Part model, mm, in its own coordinate system. Face numbers are marked on the shaded views. A direction names the side the tool comes from. Coordinates: 2 decimals unless noted, no trailing zeros. Order: outer loops, then holes, each group sorted by start corner. A loop starts at its lowest first (then second) coordinate and runs counter-clockwise, first axis right, second up.
from build123d import *

# Parameters (mm, degrees)
SKETCH1_W                  = 43.18
SKETCH1_H                  = 50.927
BOSS_EXTRUDE1_DEPTH        = 5.08
BOSS_EXTRUDE2_DEPTH        = 2.286
BOSS_EXTRUDE3_DEPTH        = 2.286
SKETCH4_W                  = 43.18
SKETCH4_H                  = 50.927
CUT_EXTRUDE1_DEPTH         = 2.794
BOSS_EXTRUDE4_DEPTH        = 2.54
SKETCH6_W                  = 63.373
SKETCH6_H                  = 2.286
BOSS_EXTRUDE5_DEPTH        = 27.813
SKETCH7_W                  = 25.273
SKETCH7_H                  = 63.373
BOSS_EXTRUDE6_DEPTH        = 12.7
SKETCH8_W                  = 63.373
SKETCH8_H                  = 2.286
BOSS_EXTRUDE7_DEPTH        = 27.813
SKETCH9_W                  = 25.273
SKETCH9_H                  = 63.373
BOSS_EXTRUDE8_DEPTH        = 12.7
SKETCH10_W                 = 22.987
SKETCH10_H                 = 12.7
CUT_EXTRUDE2_DEPTH         = 70.723
SKETCH11_W                 = 22.987
SKETCH11_H                 = 12.7
CUT_EXTRUDE3_DEPTH         = 70.723
HOLE1_D                    = 4.9784
HOLE1_DEPTH                = 2.286
M3_5_CLEARANCE_HOLE1_D     = 4.1402
M3_5_CLEARANCE_HOLE1_DEPTH = 69.723
M3_5_CLEARANCE_HOLE2_D     = 4.1402
M3_5_CLEARANCE_HOLE2_DEPTH = 2.286025
M25_CLEARANCE_HOLE1_D      = 28.575
M25_CLEARANCE_HOLE1_DEPTH  = 2.286025
M6_5_CLEARANCE_HOLE1_D     = 7.1882
M6_5_CLEARANCE_HOLE1_DEPTH = 2.286025
HOLE2_D                    = 4.9784
HOLE2_DEPTH                = 2.286025
M3_5_CLEARANCE_HOLE3_D     = 4.1402
M3_5_CLEARANCE_HOLE3_DEPTH = 2.286
HOLE3_D                    = 4.9784
HOLE3_DEPTH                = 2.28605
M3_5_CLEARANCE_HOLE4_D     = 4.1402
M3_5_CLEARANCE_HOLE4_DEPTH = 14.98605
CHAMFER1_SIZE2             = 0.596085437
CHAMFER1_SIZE              = 2.159
CHAMFER2_SIZE              = 2.159
CHAMFER3_SIZE              = 2.159
CHAMFER3_SIZE2             = 0.596085437
FILLET1_R                  = 0.8128
FILLET2_R                  = 1.6256
FILLET3_R                  = 3.0988


with BuildPart() as part:
    # Sketch1 → Boss-Extrude1 (new body)
    with BuildSketch(Plane.XY.offset(2.286)):
        with Locations((1.27, 0)):
            Rectangle(SKETCH1_W, SKETCH1_H)
    extrude(amount=-BOSS_EXTRUDE1_DEPTH)

    # Sketch2 → Boss-Extrude2 (add)
    with BuildSketch(Plane(origin=(0, 25.4635, 0), x_dir=(-1, 0, 0), z_dir=(0, 1, 0))):
        Polygon((20.32, 2.286), (20.32, -67.437), (-22.86, -2.794), (-22.86, 2.286), align=None)
    extrude(amount=BOSS_EXTRUDE2_DEPTH)

    # Sketch3 → Boss-Extrude3 (add)
    with BuildSketch(Plane.XZ.offset(25.4635)):
        Polygon((-20.32, -67.437), (-20.32, 2.286), (22.86, 2.286), (22.86, -2.794), align=None)
    extrude(amount=BOSS_EXTRUDE3_DEPTH)

    # Sketch4 → Cut-Extrude1 (cut)
    with BuildSketch(Plane(origin=(0, 0, -2.794), x_dir=(-1, 0, 0), z_dir=(0, 0, -1))):
        with Locations((-1.27, 0)):
            Rectangle(SKETCH4_W, SKETCH4_H)
    extrude(amount=-CUT_EXTRUDE1_DEPTH, mode=Mode.SUBTRACT)

    # Sketch5 → Boss-Extrude4 (add)
    with BuildSketch(Plane.ZY.offset(20.32)):
        Polygon((-67.437, -25.4635), (0, -25.4635), (0, 25.4635), (-67.437, 25.4635), (-67.437, 27.7495), (2.286, 27.7495), (2.286, -27.7495), (-67.437, -27.7495), align=None)
    extrude(amount=BOSS_EXTRUDE4_DEPTH)

    # Sketch6 → Boss-Extrude5 (add)
    with BuildSketch(Plane.ZY.offset(22.86)):
        with Locations((-35.7505, 26.6065)):
            Rectangle(SKETCH6_W, SKETCH6_H)
    extrude(amount=BOSS_EXTRUDE5_DEPTH)

    # Sketch7 → Boss-Extrude6 (add)
    with BuildSketch(Plane.XZ.offset(-25.4635)):
        with Locations((-38.0365, -35.7505)):
            Rectangle(SKETCH7_W, SKETCH7_H)
    extrude(amount=BOSS_EXTRUDE6_DEPTH)

    # Sketch8 → Boss-Extrude7 (add)
    with BuildSketch(Plane.ZY.offset(22.86)):
        with Locations((-35.7505, -26.6065)):
            Rectangle(SKETCH8_W, SKETCH8_H)
    extrude(amount=BOSS_EXTRUDE7_DEPTH)

    # Sketch9 → Boss-Extrude8 (add)
    with BuildSketch(Plane(origin=(0, -25.4635, 0), x_dir=(-1, 0, 0), z_dir=(0, 1, 0))):
        with Locations((38.0365, -35.7505)):
            Rectangle(SKETCH9_W, SKETCH9_H)
    extrude(amount=BOSS_EXTRUDE8_DEPTH)

    # Sketch10 → Cut-Extrude2 (cut, through all)
    with BuildSketch(Plane(origin=(0, 0, -67.437), x_dir=(-1, 0, 0), z_dir=(0, 0, -1))):
        with Locations((39.1795, 21.3995)):
            Rectangle(SKETCH10_W, SKETCH10_H)
    extrude(amount=-CUT_EXTRUDE2_DEPTH, mode=Mode.SUBTRACT)

    # Sketch11 → Cut-Extrude3 (cut, through all)
    with BuildSketch(Plane(origin=(0, 0, -67.437), x_dir=(-1, 0, 0), z_dir=(0, 0, -1))):
        with Locations((39.1795, -21.3995)):
            Rectangle(SKETCH11_W, SKETCH11_H)
    extrude(amount=-CUT_EXTRUDE3_DEPTH, mode=Mode.SUBTRACT)

    # Hole1
    with Locations(Plane(origin=(0, -27.7495, 0), x_dir=(-1, 0, 0), z_dir=(0, -1, 0))):
        with Locations((12.7, 10.1854), (-12.7, 10.1854), (12.7, 42.3164)):
            Hole(HOLE1_D / 2, depth=HOLE1_DEPTH)

    # M3.5 Clearance Hole1
    with Locations(Plane.XY.offset(2.286)):
        with Locations((0, -18.415)):
            Hole(M3_5_CLEARANCE_HOLE1_D / 2, depth=M3_5_CLEARANCE_HOLE1_DEPTH)

    # M3.5 Clearance Hole2
    with Locations(Plane(origin=(0, 0, 0), x_dir=(-1, 0, 0), z_dir=(0, 0, -1))):
        with Locations((-18.415, 0), (18.415, 0), (0, 18.415)):
            Hole(M3_5_CLEARANCE_HOLE2_D / 2, depth=M3_5_CLEARANCE_HOLE2_DEPTH)

    # M25 Clearance Hole1
    with Locations(Plane(origin=(0, 0, 0), x_dir=(-1, 0, 0), z_dir=(0, 0, -1))):
        with Locations((0, 0)):
            Hole(M25_CLEARANCE_HOLE1_D / 2, depth=M25_CLEARANCE_HOLE1_DEPTH)

    # M6.5 Clearance Hole1
    with Locations(Plane(origin=(0, 0, 0), x_dir=(-1, 0, 0), z_dir=(0, 0, -1))):
        with Locations((17.5, 17.5), (-17.5, -17.5)):
            Hole(M6_5_CLEARANCE_HOLE1_D / 2, depth=M6_5_CLEARANCE_HOLE1_DEPTH)

    # Hole2
    with Locations(Plane(origin=(0, 0, 0), x_dir=(-1, 0, 0), z_dir=(0, 0, -1))):
        with Locations((17.960512242, -17.960512242), (-17.960512242, 17.960512242)):
            Hole(HOLE2_D / 2, depth=HOLE2_DEPTH)

    # M3.5 Clearance Hole3
    with Locations(Plane(origin=(0, -15.0495, 0), x_dir=(-1, 0, 0), z_dir=(0, -1, 0))):
        with Locations((38.1, 61.214), (38.1, 48.514), (38.1, 35.814), (38.1, 23.114), (38.1, 10.414)):
            Hole(M3_5_CLEARANCE_HOLE3_D / 2, depth=M3_5_CLEARANCE_HOLE3_DEPTH)

    # Hole3
    with Locations(Plane(origin=(0, 25.4635, 0), x_dir=(-1, 0, 0), z_dir=(0, -1, 0))):
        with Locations((12.7, 10.1854), (-12.7, 10.1854), (12.7, 42.3164)):
            Hole(HOLE3_D / 2, depth=HOLE3_DEPTH)

    # M3.5 Clearance Hole4
    with Locations(Plane(origin=(0, 12.7635, 0), x_dir=(-1, 0, 0), z_dir=(0, -1, 0))):
        with Locations((38.1, 61.214), (38.1, 48.514), (38.1, 35.814), (38.1, 23.114), (38.1, 10.414)):
            Hole(M3_5_CLEARANCE_HOLE4_D / 2, depth=M3_5_CLEARANCE_HOLE4_DEPTH)

    # Chamfer1
    chamfer1_edges = [part.edges().sort_by_distance(p)[0] for p in [
        (-20.32, 26.6065, -67.437),
    ]]
    chamfer(chamfer1_edges, length=CHAMFER1_SIZE, length2=CHAMFER1_SIZE2)

    # Chamfer2
    chamfer2_edges = [part.edges().sort_by_distance(p)[0] for p in [
        (-50.673, -13.9065, -67.437),
        (-50.673, 13.9065, -67.437),
        (-50.673, -13.9065, -4.064),
        (-50.673, 13.9065, -4.064),
    ]]
    chamfer(chamfer2_edges, length=CHAMFER2_SIZE)

    # Chamfer3
    chamfer3_edges = [part.edges().sort_by_distance(p)[0] for p in [
        (-20.32, -26.6065, -67.437),
    ]]
    chamfer3_side = [part.faces().sort_by_distance(p)[0] for p in [
        (1.27, -26.6065, -35.1155),
    ]]
    chamfer(chamfer3_edges, length=CHAMFER3_SIZE, length2=CHAMFER3_SIZE2, reference=chamfer3_side[0])

    # Fillet1
    fillet1_edges = [part.edges().sort_by_distance(p)[0] for p in [
        (0, -25.4635, 0),
        (-25.4, 25.4635, -35.7505),
        (-25.4, -25.4635, -35.7505),
        (-27.686, -15.0495, -35.7505),
        (-27.686, 15.0495, -35.7505),
        (0, 25.4635, 0),
    ]]
    fillet(fillet1_edges, radius=FILLET1_R)

    # Fillet2
    fillet2_edges = [part.edges().sort_by_distance(p)[0] for p in [
        (-22.86, -26.6065, -4.064),
        (-22.86, 26.6065, -4.064),
    ]]
    fillet(fillet2_edges, radius=FILLET2_R)

    # Fillet3
    fillet3_edges = [part.edges().sort_by_distance(p)[0] for p in [
        (0, 27.7495, 2.286),
        (-27.686, -27.7495, -35.7505),
        (0, -27.7495, 2.286),
        (-25.4, 12.7635, -35.7505),
        (-25.4, -12.7635, -35.7505),
        (-27.686, 27.7495, -35.7505),
    ]]
    fillet(fillet3_edges, radius=FILLET3_R)


solid = part.part
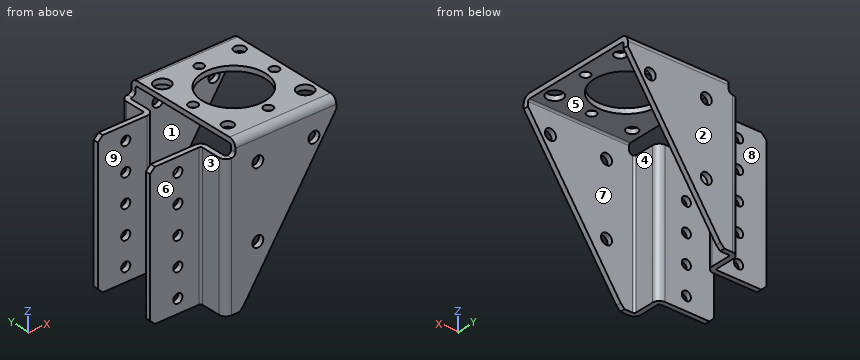
Q1. Which spindle directions (+Z, -Z, +X, -X, +Y, -Y) get a long thin tool onto all of the face, cutting with end or side? Do the marked faces 5, 6, 7, 8 and 9. Say none if no direction does.
Results list:
face 5: -Z, +X, -X
face 6: +Z, -Z, -X, -Y
face 7: -Z, +X
face 8: +Z, -Z, -X, +Y
face 9: +Z, -Z, +X, -X
Q2. Cut at D-D on x = 17.5. Write the cut outline in (y, z), and give its area (3 significant figures).
Results list:
outline: (-27.75, -10.82) - (-25.46, -10.82) - (-25.46, -0.81) arc R0.81 cw to (-24.65, 0) - (-21.09, 0) - (-21.09, 2.29) - (-24.65, 2.29) arc R3.1 ccw to (-27.75, -0.81) - close; (-13.91, 0) - (-1.86, 0) - (-1.86, 2.29) - (-13.91, 2.29) - close; (1.86, 0) - (15.51, 0) - (15.51, 2.29) - (1.86, 2.29) - close; (20.41, 0) - (24.65, 0) arc R0.81 cw to (25.46, -0.81) - (25.46, -10.82) - (27.75, -10.82) - (27.75, -0.81) arc R3.1 ccw to (24.65, 2.29) - (20.41, 2.29) - close
area: 136 mm2
Q3. Wall check: line 1 along Y through (x, z) = (-13, -2); line 2 along Y through (x, z) = (-31, -62.5); line 3 along Y through (x, z) = (-17.5, 1.5). Give the ranges that are in metal, low to high.
Results list:
line 1: y = -27.75 to -25.46, 25.46 to 27.75
line 2: y = -15.05 to -12.76, 12.76 to 15.05
line 3: y = -26.71 to -20.41, -15.51 to -1.86, 1.86 to 13.91, 21.09 to 26.71
Q4. Cut at B-B on x = -34.5. Write the cut outline in (y, z), and give its area (3 significant figures).
Results list:
outline: (-15.05, -67.44) - (-12.76, -67.44) - (-12.76, -4.06) - (-15.05, -4.06) - close; (12.76, -67.44) - (15.05, -67.44) - (15.05, -4.06) - (12.76, -4.06) - close
area: 290 mm2
Q5. Pin check, flat tips, straight feed: pin 1 Ø6.5 at (x, z) = (-42, -45.5) entering from +Y; pin 2 Ø4.5 at (x, z) = (-12.7, -10.19) entering from -Y; pin 3 Ø10 at (x, y) = (-11.5, -16) entering from -Z; pin 4 Ø1 at (y, z) = (-20.5, -52) entering from -X. Stop position of each tip, or through.
Results list:
pin 1: stops at y = 15.05
pin 2: passes through
pin 3: stops at z = 0
pin 4: stops at x = -27.69
Q6. Mould opens along Y. For the marked faces 1, 2, 3 and 4 say: pulls with the +Y half, pulls with the -Y half, needs draft (parallel to the pull), parting line crosses it, or undercut.
Results list:
face 1: undercut
face 2: pulls with the +Y half
face 3: needs draft
face 4: undercut
Q7. Cut at C-C on y = -6. Write the cut outline in (x, z).
Results list:
outline: (-22.86, 0) - (-12.97, 0) - (-12.97, 2.29) - (-22.86, 2.29) - close; (12.97, 0) - (22.86, 0) - (22.86, 2.29) - (12.97, 2.29) - close
Q8. Cut at A-A on y = 0. Write the cut outline in (x, z), and give its area (3 significant figures).
Results list:
outline: (-22.86, 0) - (-20.49, 0) - (-20.49, 2.29) - (-22.86, 2.29) - close; (-16.34, 0) - (-14.29, 0) - (-14.29, 2.29) - (-16.34, 2.29) - close; (14.29, 0) - (16.34, 0) - (16.34, 2.29) - (14.29, 2.29) - close; (20.49, 0) - (22.86, 0) - (22.86, 2.29) - (20.49, 2.29) - close
area: 20.3 mm2
